Read the model definition and answer for the solid it produces. Units are mm, in the model's axes. Give positions to 0.01 mm unless a question says otherwise; leave off trailing zeros. Write each loop counter-clockwise with the first axis right and the second up, starting at its lowest first coordinate (ties: lowest second). Pieces come first, ordered by that corner, then holes. Notation, with made-up numbers: (6, -18.5) - (37, -18.5) arc R17 ccw to (37, -9.5) - close; hole circle Ø4 at (85.5, 65.5). An arc over 180 degrees is marked (long way). Answer as CSV lines item,"result".
```python
from build123d import *

# Parameters (mm, degrees)
F0_W     = 76.2
F0_H     = 342.9
F1_DEPTH = 25.4
F3_D     = 5
F3_DEPTH = 79.1972
F3_TIP   = 1.5021515476
F5_D     = 5
F5_DEPTH = 79.1972
F5_TIP   = 1.5021515476


with BuildPart() as f1:
    # F0 (on Front) → F1 (new body)
    with BuildSketch(Plane.XZ):
        with Locations((38.1, 171.45)):
            Rectangle(F0_W, F0_H)
    extrude(amount=F1_DEPTH)

    # F3
    with Locations(Plane.XY.offset(342.9)):
        with Locations((63.5, -12.7)):
            Hole(F3_D / 2, depth=F3_DEPTH)
            with Locations((0, 0, -(F3_DEPTH + F3_TIP / 2))):  # 118° drill point
                Cone(0, F3_D / 2, F3_TIP, mode=Mode.SUBTRACT)

    # F5
    with Locations(Plane(origin=(0, 0, 0), x_dir=(1, 0, 0), z_dir=(0, 0, -1))):
        with Locations((57.15, 12.7), (19.05, 12.7)):
            Hole(F5_D / 2, depth=F5_DEPTH)
            with Locations((0, 0, -(F5_DEPTH + F5_TIP / 2))):  # 118° drill point
                Cone(0, F5_D / 2, F5_TIP, mode=Mode.SUBTRACT)


solid = f1.part
```
(1) A cutting plane is placed at A-A (z = 30). Write down the section's boundary in (x, y), and give its area (3 significant figures).
Worked out:
outline,"(0, -25.4) - (76.2, -25.4) - (76.2, 0) - (0, 0) - close; hole circle Ø5 at (19.05, -12.7); hole circle Ø5 at (57.15, -12.7)"
area,"1,900 mm^2"
(2) This flat-tipped pin is pushed along its axis until it touches: P1, Ø12, axis at x = 43.5, z = 297, coming from the +Y side. Where does it stop, or does it pass through?
Worked out:
P1,"stops at y = 0"
(3) Find the intervals of material crossed by L1, parallel to X at y = -12.7, z = 54.5; L2, parallel to Y at x = 57.15, z = 48.5; L3, parallel to Y at x = 63, z = 326, in increasing order.
Worked out:
L1,"x = 0 to 16.55, 21.55 to 54.65, 59.65 to 76.2"
L2,"y = -25.4 to -15.2, -10.2 to 0"
L3,"y = -25.4 to -15.15, -10.25 to 0"
